The listing builds one solid part. Answer for the finished solid, in the listing's coordinates (mm). Face numbers are marked on the shaded views. A direction names the side the tool comes from. Round coordinates to 2 decimals unless told otherwise and drop trailing zeros. Order: outer loops, then holes, each group sorted by start corner. A loop starts at its lowest first (then second) coordinate and runs counter-clockwise, first axis right, second up. Notation, with made-up numbers: (79, 29.25) -> (86, 29.25) arc R35 ccw to (86, 62.25) -> close; hole circle Ø4 at (79.5, 63). An arc over 180 degrees is marked (long way). Return JSON: item names as keys, results as strings. Group by question number.
(1) Each of these flat-tipped pins is pushed along its axis until it touches: pin 1 (6 mm diameter, centred on y = 26, z = -89, fed in from -X); pin 2 (1 mm diameter, centred on x = 1.5, z = -50, fed in from +Y); pin 3 (1.5 mm diameter, centred on x = 0.5, z = -70, fed in from +Y); pin 4 (2.5 mm diameter, centred on x = 0, y = 35.75, fed in from +Z). Where does it stop, or does it pass through?
(2) The part is cut by section A-A (z = -40). Determine the outline of the cut face in (x, y).
(3) Which of the six approach directions +Z, -Z, +X, -X, +Y, -Y give full straight-line access (tool end or side, diameter ignored) to the marked faces 1 and 2?
(4) Consider line 1 (X direction, y = 35.75, z = -117.75); line 2 (Y direction, x = 0, z = -115). Determine where each line is inside the solid, lowest interval first. Write a range as [from, to].
Autodesk Inventor part; units mm, degrees
ref_plane "YZ Plane" through (0, 0, 0) normal (1, 0, 0) x (0, 1, 0)
ref_plane "XZ Plane" through (0, 0, 0) normal (0, 1, 0) x (-1, 0, 0)
ref_plane "XY Plane" through (0, 0, 0) normal (0, 0, 1) x (1, 0, 0)
sketch "Sketch1" plane through (0, 0, 0) normal (0, 0, 1) x (1, 0, 0)
  circle A0 centre (0, 0) radius 2.5
  dimension "d0" = 5
sketch "Sketch2" plane through (0, 0, 0) normal (1, 0, 0) x (0, 1, 0)
  line L0 (0, 0) -> (0, -72.5029)
  line L1 (2.6789, -78.248) -> (33.0711, -103.752)
  line L2 (35.75, -109.4971) -> (35.75, -123)
  arc A0 (0, -72.5029) -> (2.6789, -78.248) centre (7.5, -72.5029) ccw
  arc A1 (35.75, -109.4971) -> (33.0711, -103.752) centre (28.25, -109.4971) ccw
  point P0 (0, -76)
  point P1 (35.75, -106)
  dimension "d1" = 76
  dimension "d2" = 35.75
  dimension "d3" = 17
  dimension "d4" = 30
  dimension "d5" = 7.5
sweep "Sweep1" add profiles "Sketch1" path "Sketch2"
shell "Shell1" thickness 0.5 removed faces 2 at (-0.852, 0.5526, 0) at (0.4229, 36.3026, -123)
properties part number "158 diameter 76" material "Iron, Gray"
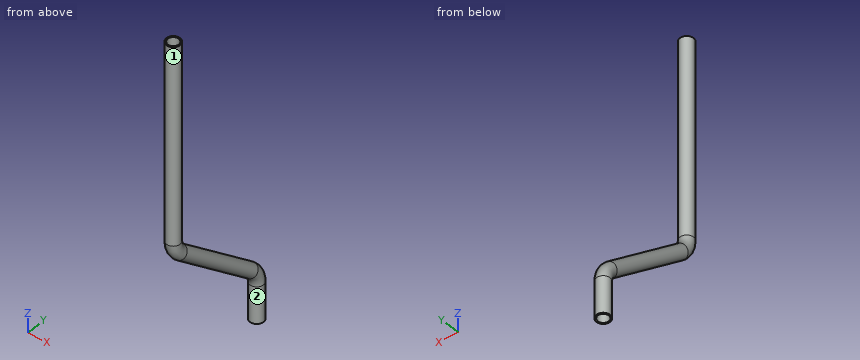
Answer below:
{
 "1": {"pin 1": "passes through", "pin 2": "stops at y = 2.29", "pin 3": "stops at y = 2.5", "pin 4": "stops at z = -101.69"},
 "2": {"outline": "circle Ø5 at (0, 0); hole circle Ø4 at (0, 0)"},
 "3": {"face 1": "+Z", "face 2": "-Z"},
 "4": {"line 1": "x = [-2.5, -2], [2, 2.5]", "line 2": "y = [33.25, 33.75], [37.75, 38.25]"}
}
